Source: CAD feature listing. Evaluate the final solid. Frame: model axes, mm. A direction names the side the tool comes from. Coordinates: 2 decimals unless noted, no trailing zeros. Write each loop counter-clockwise with the first axis right and the second up, starting at its lowest first coordinate (ties: lowest second). Pieces come first, ordered by that corner, then holes. Notation, with made-up numbers: (24.5, -2.75) - (38.5, -2.75) arc R24 ccw to (38.5, 19.25) - close; hole circle Ø2 at (51, -23). An arc over 180 degrees is marked (long way). One line per question, with ' | ' between items. Start each with the question number.
Q1. Cut plane C-C, the plane x = 56. Return loops of the section in (y, z), plus the area to 3 significant figures.
Q2. Line query: line 1 (X direction, y = -3, z = 3.15); line 2 (Y direction, x = 48.5, z = 2.3); line 3 (Y direction, x = -20, z = 3.15). Output: solid intervals per line, ascending.
Q3. Access query for faces 1 (the face through (-1, 1, 0)), 2 (the face through (-40, 5, 3)). Directions: +Z, -Z, +X, -X, +Y, -Y. A direction counts if a zero-diameter tool reaches every point of the face in a straight line with its end or side. Return the directions, or none.
Q4. Draft query along X for faces 3 (the face through (36, 15.5, 3)), 4 (the face through (-29, -10, 3)), 5 (the face through (-70, -1, 2)), 6 (the face through (-1, -50, 2)). Return one class per face: +X half, -X half, draft (parallel to the pull), parting line (faces both ways), or undercut.
Q5. Cut plane A-A, the plane x = -25. Return loops of the section in (y, z).
Q6. Cut plane B-B, the plane z = 1.4. Return loops of the section in (x, y), plus the area to 3 significant figures.
Q7. Contact query for a flat-ended pin moving along its axis: P1, Ø1.8, axis at x = 56, y = 5.5, coming from the -Z side. Output: stop coordinate, or through.
```python
from build123d import *

# Parameters (mm, degrees)
SKIZZE1_W                       = 140
SKIZZE1_H                       = 100
AUFSATZ_LINEAR_AUSTRAGEN1_DEPTH = 5
SKIZZE2_W                       = 22
SKIZZE2_H                       = 31
SCHNITT_LINEAR_AUSTRAGEN1_DEPTH = 87.168439698
SKIZZE4_R                       = 1.5
SKIZZE4_W                       = 28
SKIZZE4_H                       = 20
SCHNITT_LINEAR_AUSTRAGEN3_DEPTH = 87.168439698
SKIZZE3_R                       = 0.5
SCHNITT_LINEAR_AUSTRAGEN2_DEPTH = 87.168439698


with BuildPart() as part:
    # Skizze1 → Aufsatz-Linear austragen1 (new body)
    with BuildSketch(Plane.XY):
        Rectangle(SKIZZE1_W, SKIZZE1_H)
    extrude(amount=AUFSATZ_LINEAR_AUSTRAGEN1_DEPTH)

    # Skizze2 → Schnitt-Linear austragen1 (cut, through all)
    with BuildSketch(Plane.XY.offset(5)):
        with Locations((-29, 5.5)):
            Rectangle(SKIZZE2_W, SKIZZE2_H)
    extrude(amount=-SCHNITT_LINEAR_AUSTRAGEN1_DEPTH, mode=Mode.SUBTRACT)

    # Skizze4 → Schnitt-Linear austragen3 (cut, through all)
    with BuildSketch(Plane.XY.offset(5)):
        with Locations((16, 5.5)):
            Circle(SKIZZE4_R)
        with Locations((56, 5.5)):
            Circle(SKIZZE4_R)
        with Locations((36, 5.5)):
            Rectangle(SKIZZE4_W, SKIZZE4_H)
    extrude(amount=-SCHNITT_LINEAR_AUSTRAGEN3_DEPTH, mode=Mode.SUBTRACT)

    # Skizze3 → Schnitt-Linear austragen2 (cut, through all)
    with BuildSketch(Plane.XY.offset(5)):
        with Locations((-40, 21)):
            Circle(SKIZZE3_R)
        with Locations((-18, 21)):
            Circle(SKIZZE3_R)
        with Locations((-18, -10)):
            Circle(SKIZZE3_R)
        with Locations((-40, -10)):
            Circle(SKIZZE3_R)
        with Locations((22, 15.5)):
            Circle(SKIZZE3_R)
        with Locations((50, 15.5)):
            Circle(SKIZZE3_R)
        with Locations((50, -4.5)):
            Circle(SKIZZE3_R)
        with Locations((22, -4.5)):
            Circle(SKIZZE3_R)
    extrude(amount=-SCHNITT_LINEAR_AUSTRAGEN2_DEPTH, mode=Mode.SUBTRACT)


solid = part.part
```
Reply:
1) outline: (-50, 0) - (4, 0) - (4, 5) - (-50, 5) - close; (7, 0) - (50, 0) - (50, 5) - (7, 5) - close | area: 485 mm^2
2) line 1: x = -70 to -40, -18 to 22, 50 to 70 | line 2: y = -50 to -4.5, 15.5 to 50 | line 3: y = -50 to -10, 21 to 50
3) face 1: -Z, +X, -X, +Y, -Y | face 2: +Z, -Z
4) face 3: undercut | face 4: undercut | face 5: -X half | face 6: draft
5) outline: (-50, 0) - (-10, 0) - (-10, 5) - (-50, 5) - close; (21, 0) - (50, 0) - (50, 5) - (21, 5) - close
6) outline: (-70, -50) - (70, -50) - (70, 50) - (-70, 50) - close; hole (-40, -9.5) arc R0.5 ccw (long way) to (-39.5, -10) - (-18.5, -10) arc R0.5 ccw (long way) to (-18, -9.5) - (-18, 20.5) arc R0.5 ccw (long way) to (-18.5, 21) - (-39.5, 21) arc R0.5 ccw (long way) to (-40, 20.5) - close; hole circle Ø3 at (16, 5.5); hole (22, -4) arc R0.5 ccw (long way) to (22.5, -4.5) - (49.5, -4.5) arc R0.5 ccw (long way) to (50, -4) - (50, 15) arc R0.5 ccw (long way) to (49.5, 15.5) - (22.5, 15.5) arc R0.5 ccw (long way) to (22, 15) - close; hole circle Ø3 at (56, 5.5) | area: 12,700 mm^2
7) P1: passes through
